Solid Edge part; units mm, degrees
sketch "Sketch1" plane through (0, 0, 0) normal (1, 0, 0) x (0, 1, 0)
  line L0 (-30.361, 27.2865) -> (-15.361, 27.2865)
  line L1 (-15.361, 27.2865) -> (-15.361, 13.2865)
  line L2 (-15.361, 13.2865) -> (-30.361, 13.2865)
  line L3 (-30.361, 13.2865) -> (-30.361, 27.2865)
  dimension "D1" = 30.361
  dimension "D2" = 15.361
extrude "Protrusion1" add sketch "Sketch1" against normal blind 15
sketch "Sketch2" plane through (0, -22.861, 20.2865) normal (1, 0, 0) x (0, 1, 0)
  line L0 (-7.5, 6) -> (-6.5, 6)
  line L1 (-6.5, 6) -> (-6.5, -6)
  line L2 (-6.5, -6) -> (-7.5, -6)
  line L3 (-7.5, -6) -> (-7.5, 6)
  dimension "D1" = 7.5
extrude "Cutout1" cut sketch "Sketch2" against normal through all
chamfer "afschuin9x4" distance 9 distance2 4 1 edges at (0, -15.361, 20.2865) measured on face at (0, -18.011, 25.0932)
chamfer "Chamfer_4" distance 9 distance2 2 1 edges at (-15, -15.361, 20.2865) measured on face at (-15, -18.011, 25.0932)
hole "schroefdraadM4" at (-7.5, -29.361, 20.2865) direction (0, 1, 0) diameter 3.242 depth 11 tip angle 118 thread major 4 thread length 7
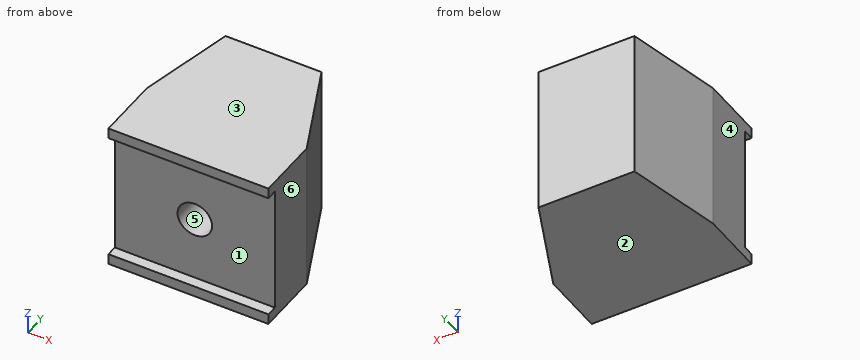
Read the model definition and answer for the solid it produces. Units are mm, in the model's axes. Face numbers are marked on the shaded views. A direction names the side the tool comes from. Give positions to 0.01 mm unless a question says otherwise; leave off trailing zeros. Loops run counter-clockwise (first coordinate to the right, second up) from the corner with the lowest first, then second, coordinate; pieces in that order, holes last.
Item 1: For the marked faces 5 and 6, determine the directions among +Z, -Z, +X, -X, +Y, -Y from which every point of the face is accessible in a straight line to the end or side of a thin tool.
Item 2: The part is cut by section A-A (x = -12.25). Write down the section's boundary in (y, z).
Item 3: The part is cut by section B-B (y = -28.5). Write down the section's boundary in (x, z), and give its area (3 significant figures).
Item 4: The part is cut by section D-D (y = -22.25). Write down the section's boundary in (x, z), and give its area (3 significant figures).
Item 5: Each of these flat-tipped pins is pushed along its axis until it touches: pin 1 Ø1.5 at (x, z) = (-10, 17.5) entering from -Y; pin 2 Ø1.5 at (y, z) = (-17, 16) entering from +X; pin 3 Ø1.5 at (y, z) = (-18, 24) entering from -X. Where does it stop, or does it pass through?
Item 6: The mould has two halves that part along Z. Classify the marked faces 1, 2, 3 and 4: released by +Z, released by -Z, zero draft, split by the parting line, or undercut.
Item 7: The part is cut by section C-C (z = 18). Write down the section's boundary in (x, y), and give its area (3 significant figures).
Item 8: Find the intervals of material crossed by line 1 along Z through (x, y) = (-7.5, -25.75); line 2 along Y through (x, z) = (-10.5, 24.75); line 3 along Z through (x, y) = (-8.5, -20.75), in increasing order.
Taken from the geometry:
1. face 5: -Y
1. face 6: +Z, -Z, +X, +Y, -Y
2. outline: (-30.36, 13.29) - (-15.36, 13.29) - (-15.36, 27.29) - (-30.36, 27.29) - (-30.36, 26.29) - (-29.36, 26.29) - (-29.36, 14.29) - (-30.36, 14.29) - close
3. outline: (-15, 13.29) - (0, 13.29) - (0, 27.29) - (-15, 27.29) - close; hole circle Ø3.24 at (-7.5, 20.29)
3. area: 202 mm2
4. outline: (-14.53, 13.29) - (-0.94, 13.29) - (-0.94, 27.29) - (-14.53, 27.29) - close; hole circle Ø3.24 at (-7.5, 20.29)
4. area: 182 mm2
5. pin 1: stops at y = -29.36
5. pin 2: stops at x = -2.94
5. pin 3: stops at x = -13.75
6. face 1: undercut
6. face 2: released by -Z
6. face 3: released by +Z
6. face 4: zero draft
7. outline: (-15, -29.36) - (0, -29.36) - (0, -24.36) - (-4, -15.36) - (-13, -15.36) - (-15, -24.36) - close
7. area: 183 mm2
8. line 1: z = 13.29 to 18.67, 21.91 to 27.29
8. line 2: y = -29.36 to -15.36
8. line 3: z = 13.29 to 19.01, 21.56 to 27.29
